Could you check a few things on this drawing? It's one solid part, dimensions in mm from its lowest x, y, z. A direction names the side the tool comes from. Round coordinates to 2 decimals unless told otherwise and drop trailing zeros. Write each loop counter-clockwise with the first axis right and the second up, starting at its lowest first coordinate (ties: lowest second). Pieces come first, ordered by that corner, then holes. Notation, with made-up numbers: (43.5, 62.5) -> (75.5, 62.5) arc R21 cw to (75.5, 98.5) -> close; hole circle Ø7 at (-28, 40.25). An arc over 180 degrees is marked (long way). Answer as CSV lines item,"result".
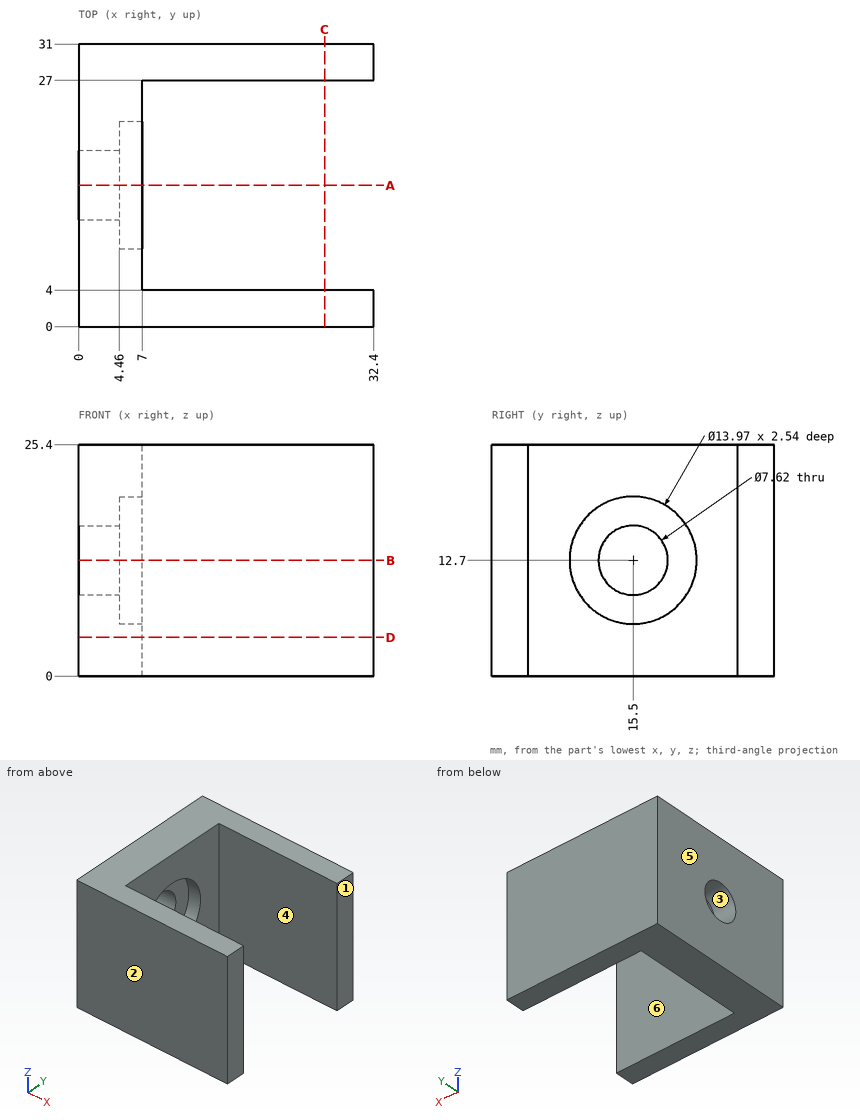
1. If we mould it in two halves opening along Y, with no side actions, what happens to the marked faces 1, 2, 3 and 4? For each: released by +Y, released by -Y, zero draft, split by the parting line, or undercut.
Numbers:
face 1,"zero draft"
face 2,"released by -Y"
face 3,"undercut"
face 4,"undercut"
2. Suppose I cut it at B-B on z = 12.7. Please give me the cut outline in (x, y) (3 decimals).
Numbers:
outline,"(0, 0) -> (32.4, 0) -> (32.4, 4) -> (7, 4) -> (7, 8.515) -> (4.46, 8.515) -> (4.46, 11.69) -> (0, 11.69) -> close; (0, 19.31) -> (4.46, 19.31) -> (4.46, 22.485) -> (7, 22.485) -> (7, 27) -> (32.4, 27) -> (32.4, 31) -> (0, 31) -> close"
3. If I drill on line 1 (Y direction, x = 18.5, z = 10); line 2 (X direction, y = 13, z = 23.75); line 3 (X direction, y = 12.5, z = 6.5), over which ranges is the centre line in solid material (lowest first)?
Numbers:
line 1,"y = 0 to 4, 27 to 31"
line 2,"x = 0 to 7"
line 3,"x = 0 to 4.46"
4. Suppose I cut it at A-A on y = 15.5. Please give me the cut outline in (x, z) (3 decimals), and give its area (3 significant figures).
Numbers:
outline,"(0, 0) -> (7, 0) -> (7, 5.715) -> (4.46, 5.715) -> (4.46, 8.89) -> (0, 8.89) -> close; (0, 16.51) -> (4.46, 16.51) -> (4.46, 19.685) -> (7, 19.685) -> (7, 25.4) -> (0, 25.4) -> close"
area,"108 mm^2"
5. Suppose I cut it at C-C on x = 27. Please give me the cut outline in (y, z), and give its area (3 significant figures).
Numbers:
outline,"(0, 0) -> (4, 0) -> (4, 25.4) -> (0, 25.4) -> close; (27, 0) -> (31, 0) -> (31, 25.4) -> (27, 25.4) -> close"
area,"203 mm^2"
6. For pin 1 Ø10 at (y, z) = (15.5, 12.7) entering from +X; pin 2 Ø1.5 at (y, z) = (5, 13) entering from -X; pin 3 Ø8 at (y, z) = (18, 22) entering from +X, each with a flat end and sliding along its axis, tell me the tip position at first contact or that it passes through.
Numbers:
pin 1,"stops at x = 4.46"
pin 2,"stops at x = 0"
pin 3,"stops at x = 7"
7. Suppose I cut it at D-D on z = 4.25. Please give me the cut outline in (x, y).
Numbers:
outline,"(0, 0) -> (32.4, 0) -> (32.4, 4) -> (7, 4) -> (7, 27) -> (32.4, 27) -> (32.4, 31) -> (0, 31) -> close"
8. On a 3-axis mill with a long thin cutter (end or side, diameter ignored), from which of +Z, -Z, +X, -X, +Y, -Y can I reach the whole of each face in a straight line? I mean the marked faces 5 and 6. Say none if no direction works.
Numbers:
face 5,"+Z, -Z, -X, +Y, -Y"
face 6,"+Z, -Z, +X"
